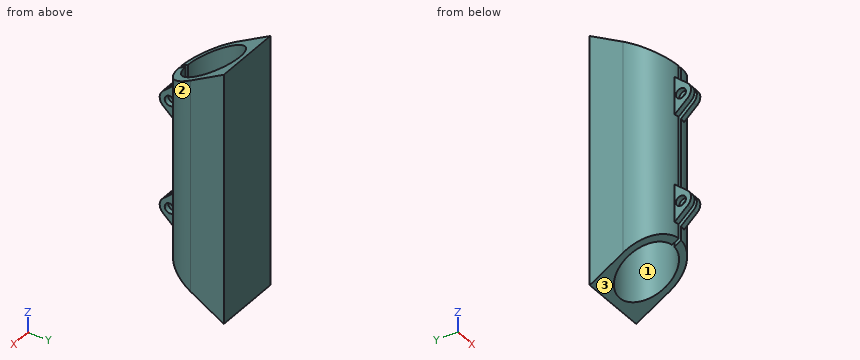
```python
from build123d import *

# Parameters (mm, degrees)
SALIENTE_EXTRUIR1_DEPTH    = 75
CROQUIS2_R                 = 1.5
SALIENTE_EXTRUIR2_DEPTH    = 2
CORTAR_EXTRUIR1_DEPTH      = 78.076531881
CORTAR_EXTRUIR1_DEPTH_BACK = 78.076531881
CROQUIS5_W                 = 1
CROQUIS5_H                 = 6.705492802
CORTAR_EXTRUIR2_DEPTH      = 78.076531881
CORTAR_EXTRUIR2_DEPTH_BACK = 78.076531881


with BuildPart() as part:
    # Croquis1 → Saliente-Extruir1 (new body)
    with BuildSketch(Plane.XY):
        with BuildLine():
            Line((-10, 10), (10, 10))
            Line((10, 10), (10, 0))
            ThreePointArc((10, 0), (7.245688373, -6.892024376), (0.5, -9.987492178))
            Line((0.5, -9.987492178), (0.5, -7.984359711))
            ThreePointArc((0.5, -7.984359711), (0, 8), (-0.5, -7.984359711))
            Line((-0.5, -7.984359711), (-0.5, -9.987492178))
            ThreePointArc((-0.5, -9.987492178), (-7.245688373, -6.892024376), (-10, 0))
            Line((-10, 0), (-10, 10))
        make_face()
    extrude(amount=SALIENTE_EXTRUIR1_DEPTH)

    # Croquis2 → Saliente-Extruir2 (add, symmetric)
    # profile 1 of 2: a face of its own
    with BuildSketch(Plane(origin=(0, 0, 0), x_dir=(0, 0, -1), z_dir=(1, 0, 0))):
        with BuildLine():
            Line((-60, -9.057857597), (-55.918368417, -13.676465368))
            ThreePointArc((-55.918368417, -13.676465368), (-53.670398363, -14.689852513), (-51.422428309, -13.676465368))
            Line((-51.422428309, -13.676465368), (-47.340796726, -9.057857597))
            Line((-47.340796726, -9.057857597), (-60, -9.057857597))
        make_face()
        with Locations((-53.670398363, -11.689852513)):
            Circle(CROQUIS2_R, mode=Mode.SUBTRACT)
    # profile 2 of 2: a face of its own
    with BuildSketch(Plane(origin=(0, 0, 0), x_dir=(0, 0, -1), z_dir=(1, 0, 0))):
        with BuildLine():
            Line((-15, -9.057857597), (-19.081631583, -13.676465368))
            ThreePointArc((-19.081631583, -13.676465368), (-21.329601637, -14.689852513), (-23.577571691, -13.676465368))
            Line((-23.577571691, -13.676465368), (-27.659203274, -9.057857597))
            Line((-27.659203274, -9.057857597), (-15, -9.057857597))
        make_face()
        with Locations(Location((-21.329601637, -11.689852513, 0), (0, 0, 180))):
            Circle(CROQUIS2_R, mode=Mode.SUBTRACT)
    extrude(amount=SALIENTE_EXTRUIR2_DEPTH, both=True)

    # Croquis5 → Cortar-Extruir1 (cut, two sides: drawn at the far end of the back side and taken through both)
    with BuildSketch(Plane.XY.offset(-CORTAR_EXTRUIR1_DEPTH_BACK)):
        with Locations((0, -11.337106112)):
            Rectangle(CROQUIS5_W, CROQUIS5_H)
    extrude(amount=CORTAR_EXTRUIR1_DEPTH + CORTAR_EXTRUIR1_DEPTH_BACK, mode=Mode.SUBTRACT)

    # Croquis6 → Cortar-Extruir2 (cut, two sides: drawn at the far end of the back side and taken through both)
    with BuildSketch(Plane(origin=(0, 0, 0), x_dir=(0, 0, -1), z_dir=(1, 0, 0)).offset(-CORTAR_EXTRUIR2_DEPTH_BACK)):
        Polygon((-75, 10), (-63.455743468, -9.987492178), (-75, -9.987492178), align=None)
        Polygon((-11.544256532, -9.987492178), (0, -9.987492178), (0, 10), align=None)
    extrude(amount=CORTAR_EXTRUIR2_DEPTH + CORTAR_EXTRUIR2_DEPTH_BACK, mode=Mode.SUBTRACT)


solid = part.part
```
Source: CAD feature listing. Evaluate the final solid. Frame: model axes, mm. Face numbers are marked on the shaded views. Give positions to 0.01 mm unless a question says otherwise; leave off trailing zeros. Loops run counter-clockwise (first coordinate to the right, second up) from the corner with the lowest first, then second, coordinate; pieces in that order, holes last. Notation, with made-up numbers: M 3.25,24 L 8.25,24 A8 cw 8.25,35 Z; hole C 74.25,19.5 d11. An arc over 180 degrees is marked long. Put each result on its own line as item: value.
Q1. Line query: probe 1 along X at (y, z) = (-13, 55.5); probe 2 along X at (y, z) = (-0.5, 13); probe 3 along Y at (x, z) = (-2.5, 50.5). Output: solid intervals per line, ascending. Write a range as [from, to].
Response values:
probe 1: x = [-2, -0.5], [0.5, 2]
probe 2: x = [-9.99, -7.98], [7.98, 9.99]
probe 3: y = [-9.68, -7.6], [7.6, 10]
Q2. Section B-B (z = 29.5). Return the cut outline in (x, y), and give its area (3 significant figures).
Response values:
outline: M -10,0 A10 ccw -0.5,-9.99 L -0.5,-7.98 A8 cw long 0.5,-7.98 L 0.5,-9.99 A10 ccw 10,0 L 10,10 L -10,10 Z
area: 154 mm²
Q3. Mould query, pull axis X, two halves, no side actions, for the marked faces 1, 2 and 3. Classes: released by +X, released by -X, zero draft, split by the parting line, or undercut.
Response values:
face 1: undercut
face 2: released by +X
face 3: zero draft
Q4. Section C-C (x = 5). Return the cut outline in (y, z) (3 decimals).
Response values:
outline: M -8.66,10.778 L -6.245,9.383 L -6.245,65.617 L -8.66,64.222 Z; M 6.245,2.169 L 10,0 L 10,75 L 6.245,72.831 Z
Q5. Section D-D (z = 17). Return the cut outline in (x, y), and give its area (3 significant figures).
Response values:
outline: M -10,0 A10 ccw -2,-9.8 L -2,-11.32 L -0.5,-11.32 L -0.5,-7.98 A8 cw long 0.5,-7.98 L 0.5,-11.32 L 2,-11.32 L 2,-9.8 A10 ccw 10,0 L 10,10 L -10,10 Z
area: 158 mm²
Q6. Section A-A (y = 2.25). Return the cut outline in (x, z).
Response values:
outline: M -10,4.48 L -7.68,4.48 L -7.68,70.52 L -10,70.52 Z; M 7.68,4.48 L 10,4.48 L 10,70.52 L 7.68,70.52 Z
Q7. Pin query (flat end, axial travel): P1, Ø5, axis at y = -11.69, z = 53.67, coming from the +X side; P2, Ø8, axis at y = -8, z = 20, coming from the -X side; P3, Ø5, axis at y = -6, z = 35.5, coming from the +X side. Return the tip coordinate at first contact, or that it passes through.
Response values:
P1: stops at x = 3.94
P2: stops at x = -9.17
P3: stops at x = 9.37
